For this review, take the finished solid that the model builds, in its own axes (mm). Round coordinates to 2 decimals unless told otherwise and drop trailing zeros. Write each loop counter-clockwise with the first axis right and the second up, starting at its lowest first coordinate (ties: lowest second). Pieces come first, ordered by that corner, then holes. Notation, with made-up numbers: (-32.75, 82.5) - (19.25, 82.5) arc R26 ccw to (19.25, 110.5) - close; hole circle Ø5 at (42, 87). An arc over 180 degrees is marked (long way). One line per item, written item: value. Start each with the question number.
Q1. Clearance check with flat-ended pins moving along their axes: pin 1 Ø6 at (x, y) = (-2.5, -7.5) entering from +Z; pin 2 Ø1 at (y, z) = (-14, 1) entering from +X; pin 3 Ø3 at (x, z) = (4.5, 0) entering from -Y. State where each tip first meets the part, or that it passes through.
Q2. For probe 1 along X at (y, z) = (-5.75, -10.25); probe 2 along Z at (x, y) = (-11.5, -18); probe 3 along Z at (x, y) = (-10.5, -16.5), list the stretches that pass through material, from the lowest coordinate up.
Q3. Add section B-B on y = -2. Write out the cut boundary in (x, z) (3 decimals).
Q4. Add section A-A on y = -22.5. Write out the cut boundary in (x, z).
```python
from build123d import *

# Parameters (mm, degrees)
F1_DEPTH = 25.4
F2_R     = 2.54


with BuildPart() as f1:
    # F0 (on Front) → F1 (new body)
    with BuildSketch(Plane.XZ):
        Polygon((-12.7, 12.7), (-12.7, -12.7), (12.7, -12.7), (12.7, -5.260512), (-5.260512, 12.7), align=None)
    extrude(amount=F1_DEPTH)

    # F2
    f2_edges = [f1.edges().sort_by_distance(p)[0] for p in [
        (-12.7, -12.7, 12.7),
        (12.7, -12.7, -5.260512),
        (-5.260512, -12.7, 12.7),
        (3.719744, 0, 3.719744),
        (3.719744, -25.4, 3.719744),
        (-8.980256, -25.4, 12.7),
        (-12.7, -25.4, 0),
        (0, -25.4, -12.7),
        (12.7, -25.4, -8.980256),
        (12.7, -12.7, -12.7),
        (12.7, 0, -8.980256),
        (-8.980256, 0, 12.7),
        (-12.7, 0, 0),
        (0, 0, -12.7),
        (-12.7, -12.7, -12.7),
    ]]
    fillet(f2_edges, radius=F2_R)


solid = f1.part
```
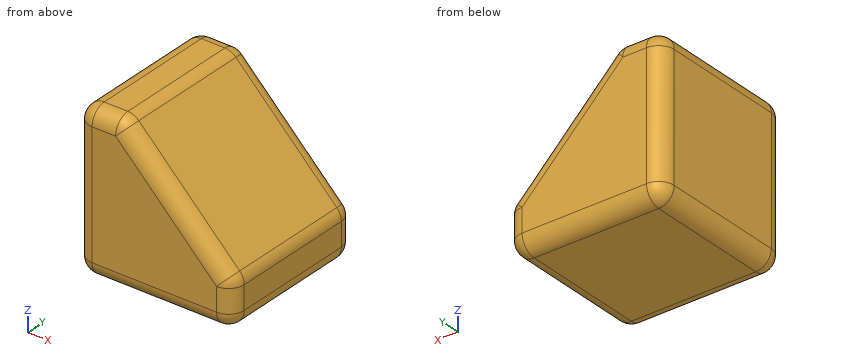
Result set:
1. pin 1: stops at z = 12.57
1. pin 2: stops at x = 6.94
1. pin 3: stops at y = -25.4
2. probe 1: x = -12.7 to 12.7
2. probe 2: z = -12.32 to 12.32
2. probe 3: z = -12.68 to 12.68
3. outline: (-12.642, -10.16) arc R2.482 ccw to (-10.16, -12.642) - (10.16, -12.642) arc R2.482 ccw to (12.642, -10.16) - (12.642, -6.313) arc R2.482 ccw to (11.915, -4.558) - (-4.558, 11.915) arc R2.482 ccw to (-6.313, 12.642) - (-10.16, 12.642) arc R2.482 ccw to (-12.642, 10.16) - close
4. outline: (-12.7, -10.16) arc R2.54 ccw to (-10.16, -12.7) - (10.16, -12.7) arc R2.54 ccw to (12.7, -10.16) - (12.7, -6.31) arc R2.54 ccw to (11.96, -4.52) - (-4.52, 11.96) arc R2.54 ccw to (-6.31, 12.7) - (-10.16, 12.7) arc R2.54 ccw to (-12.7, 10.16) - close
